```python
from build123d import *

# Parameters (mm, degrees)
SKETCH006_W     = 85.5
SKETCH006_H     = 80.5
PAD_DEPTH       = 4
SKETCH007_W     = 75.5
SKETCH007_H     = 70.5
POCKET_DEPTH    = 4.001
SKETCH014_W     = 5.5
SKETCH014_H     = 1
PAD002_DEPTH    = 2
SKETCH016_W     = 14
SKETCH016_H     = 1
PAD003_DEPTH    = 1
POCKET001_DEPTH = 3


with BuildPart() as part:
    # Sketch006 → Pad (new body)
    with BuildSketch(Plane.XY):
        Rectangle(SKETCH006_W, SKETCH006_H)
    extrude(amount=PAD_DEPTH)

    # Sketch007 (on Face6 of Pad) → Pocket (cut, through all)
    with BuildSketch(Plane.XY.offset(4)):
        Rectangle(SKETCH007_W, SKETCH007_H)
    extrude(amount=-POCKET_DEPTH, mode=Mode.SUBTRACT)

    # Sketch014 (on Face6 of Pocket) → Pad002 (join)
    with BuildSketch(Plane.XZ.offset(40.25)):
        with Locations((-16.5, 0.5)):
            Rectangle(SKETCH014_W, SKETCH014_H)
        with Locations((16.5, 0.5)):
            Rectangle(SKETCH014_W, SKETCH014_H)
    extrude(amount=PAD002_DEPTH)

    # Sketch016 (on Face1 of Pad002) → Pad003 (join)
    with BuildSketch(Plane(origin=(0, 40.25, 0), x_dir=(-1, 0, 0), z_dir=(0, 1, 0))):
        with Locations((-0.25, 0.5)):
            Rectangle(SKETCH016_W, SKETCH016_H)
    extrude(amount=PAD003_DEPTH)

    # Sketch017 (on Face2 of Pad003) → Pocket001 (cut)
    with BuildSketch(Plane(origin=(0, 40.25, 0), x_dir=(-1, 0, 0), z_dir=(0, 1, 0))):
        with BuildLine():
            ThreePointArc((-7.5, 3.5), (-8, 3), (-7.5, 2.5))
            Line((-7.5, 2.5), (7.5, 2.5))
            ThreePointArc((7.5, 2.5), (8, 3), (7.5, 3.5))
            Line((-7.5, 3.5), (7.5, 3.5))
        make_face()
    extrude(amount=-POCKET001_DEPTH, mode=Mode.SUBTRACT)


solid = part.part
```
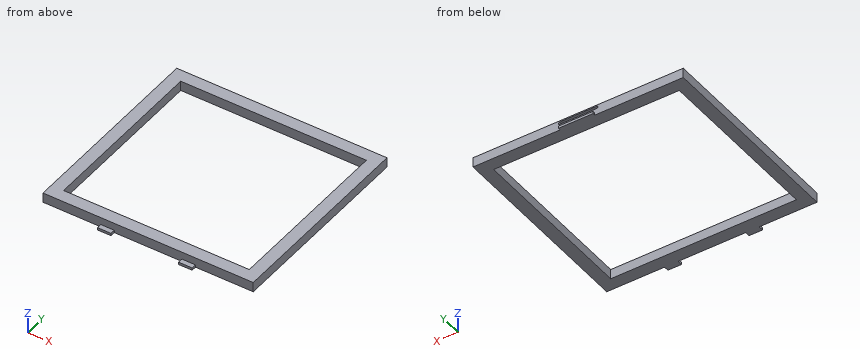
Geometry: final body of the model. Coordinates: model frame, mm. Coordinates: 2 decimals unless noted, no trailing zeros. Write each loop counter-clockwise with the first axis right and the second up, starting at its lowest first coordinate (ties: lowest second). Pieces come first, ordered by that corner, then holes. Notation, with made-up numbers: M 30.5,0 L 66.5,0 A28 cw 66.5,37 Z; hole C 29,49 d4. An arc over 180 degrees is marked long. Answer as CSV lines item,"result". Start each with the question number.
Q1. Cut plane B-B on z = 1.75. Return the cut outline in (x, y).
Q2. Cut plane C-C on y = -12. Return the cut outline in (x, z), then the cut area to 3 significant figures.
Q3. Pin query (flat end, axial travel): P1, Ø0.8, axis at x = 1, z = 3, coming from the +Y side; P2, Ø0.5, axis at y = -41, z = 0.5, coming from the -X side; P3, Ø1.6, axis at x = 17, y = -41.5, coming from the +Z side. Return the tip coordinate at first contact, or that it passes through.
Q4. Cut plane D-D on x = -16.5. Return the cut outline in (y, z).
Q5. Line query: line 1 (X direction, y = -12, z = 2.7); line 2 (Y direction, x = 16, z = 1.75); line 3 (Y direction, x = 39, z = 1.5). Output: solid intervals per line, ascending. Write a range as from..to.
Q6. Cut plane A-A on x = -35. Return the cut outline in (y, z), then the cut area to 3 significant figures.
Findings below:
1,outline,"M -42.75,-40.25 L 42.75,-40.25 L 42.75,40.25 L -42.75,40.25 Z; hole M -37.75,-35.25 L 37.75,-35.25 L 37.75,35.25 L -37.75,35.25 Z"
2,outline,"M -42.75,0 L -37.75,0 L -37.75,4 L -42.75,4 Z; M 37.75,0 L 42.75,0 L 42.75,4 L 37.75,4 Z"
2,area,"40.0 mm2"
3,P1,"stops at y = 37.25"
3,P2,"stops at x = -19.25"
3,P3,"stops at z = 1"
4,outline,"M -42.25,0 L -35.25,0 L -35.25,4 L -40.25,4 L -40.25,1 L -42.25,1 Z; M 35.25,0 L 40.25,0 L 40.25,4 L 35.25,4 Z"
5,line 1,"x = -42.75..-37.75, 37.75..42.75"
5,line 2,"y = -40.25..-35.25, 35.25..40.25"
5,line 3,"y = -40.25..40.25"
6,outline,"M -40.25,0 L -35.25,0 L -35.25,4 L -40.25,4 Z; M 35.25,0 L 40.25,0 L 40.25,4 L 35.25,4 Z"
6,area,"40.0 mm2"
